Can you work these out from the model? Positions are in its coordinate system, mm. Face numbers are marked on the shaded views. Coordinates: 2 decimals unless noted, no trailing zeros. Loops run counter-clockwise (first coordinate to the right, second up) from the corner with the lowest first, then second, coordinate; pieces in that order, holes last.
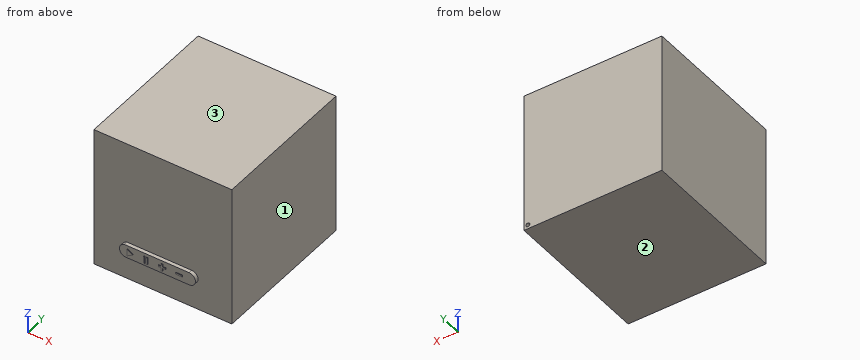
```python
from build123d import *

# Parameters (mm, degrees)
F0_W      = 93.715839088
F0_H      = 96.0587337613
F1_DEPTH  = 101.6
F2_W      = 8.2945693284
F2_H      = 8.6991842836
F2_W_2    = 8.0922637135
F2_W_3    = 8.2945674658
F2_W_4    = 7.8899562359
F3_DEPTH  = 2.54
F5_DEPTH  = 3
F6_W      = 0.9676124901
F6_H      = 4.834022373
F6_W_2    = 0.8269865066
F7_DEPTH  = 0.5
F8_W      = 1.12604897
F8_H      = 4.834022373
F9_DEPTH  = 0.5
F10_W     = 4.8627895303
F10_H     = 1.0272618383
F11_DEPTH = 0.5
F12_W     = 4.4415825978
F12_H     = 1.0272618383
F13_DEPTH = 0.5
F14_R     = 1.3332383726
F15_DEPTH = 6.35
F16_R     = 0.5696263833
F17_DEPTH = 7.62


with BuildPart() as f1:
    # F0 (on Front) → F1 (new body)
    with BuildSketch(Plane.XZ):
        with Locations((-0.6508044899, 1.3016089797)):
            Rectangle(F0_W, F0_H)
    extrude(amount=F1_DEPTH)

    # F2 (on face) → F3 (join)
    with BuildSketch(Plane.XZ.offset(101.6)):
        with BuildLine():
            Line((-19.5664688945, -20.8509583026), (-25.2310521901, -20.8509583026))
            ThreePointArc((-25.2310521901, -20.8509583026), (-28.4223170669, -25.358390925), (-24.8264390975, -29.5501425862))
            Line((-24.8264390975, -29.5501425862), (-19.5664688945, -29.5501425862))
            Line((-19.5664688945, -29.5501425862), (-19.5664688945, -20.8509583026))
        make_face()
        with Locations((-15.4191842303, -25.2005504444)):
            Rectangle(F2_W, F2_H)
        with Locations((-7.2257677093, -25.2005504444)):
            Rectangle(F2_W_2, F2_H)
        with Locations((0.9676478803, -25.2005504444)):
            Rectangle(F2_W_3, F2_H)
        with Locations((9.0599097311, -25.2005504444)):
            Rectangle(F2_W_4, F2_H)
        with BuildLine():
            Line((18.8717804849, -20.8509583026), (13.0048878491, -20.8509583026))
            Line((13.0048878491, -20.8509583026), (13.0048878491, -29.5501425862))
            Line((13.0048878491, -29.5501425862), (18.8717804849, -29.5501425862))
            ThreePointArc((18.8717804849, -29.5501425862), (23.2213726267, -25.2005504444), (18.8717804849, -20.8509583026))
        make_face()
    extrude(amount=F3_DEPTH)

    # F4 (on face) → F5 (join)
    with BuildSketch(Plane.XZ.offset(101.6)):
        Polygon((-19.0216936171, -25.3522377461), (-22.935193032, -22.9352265596), (-22.935193032, -27.7692489326), align=None)
    extrude(amount=F5_DEPTH)

    # F6 (on face) → F7 (join)
    with BuildSketch(Plane.XZ.offset(104.14)):
        with Locations((-11.4101376384, -25.3522377461)):
            Rectangle(F6_W, F6_H)
        with Locations((-9.6004614606, -25.3522377461)):
            Rectangle(F6_W_2, F6_H)
    extrude(amount=F7_DEPTH)

    # F8 (on face) → F9 (join)
    with BuildSketch(Plane.XZ.offset(104.14)):
        with Locations((0.563024485, -25.3522377461)):
            Rectangle(F8_W, F8_H)
    extrude(amount=F9_DEPTH)

    # F10 (on face) → F11 (join)
    with BuildSketch(Plane.XZ.offset(104.14)):
        with Locations((0.7227337919, -25.1438906416)):
            Rectangle(F10_W, F10_H)
    extrude(amount=F11_DEPTH)

    # F12 (on face) → F13 (join)
    with BuildSketch(Plane.XZ.offset(104.14)):
        with Locations((12.3583828099, -25.1438906416)):
            Rectangle(F12_W, F12_H)
    extrude(amount=F13_DEPTH)

    # F14 (on face) → F15 (cut)
    with BuildSketch(Plane(origin=(0, 0, 0), x_dir=(-1, 0, 0), z_dir=(0, 1, 0))):
        with Locations((-43.6146184802, -43.905235827)):
            Circle(F14_R)
    extrude(amount=-F15_DEPTH, mode=Mode.SUBTRACT)

    # F16 (on face) → F17 (cut)
    with BuildSketch(Plane(origin=(0, 0, 0), x_dir=(-1, 0, 0), z_dir=(0, 1, 0))):
        with Locations((-43.6146184802, -43.905235827)):
            Circle(F16_R)
    extrude(amount=-F17_DEPTH, mode=Mode.SUBTRACT)


solid = f1.part
```
(1) I want a section at C-C on x = -34.5. Write out the boundary of the cut face in (y, z), then the cut area to 3 significant figures.
Check values:
outline: (-101.6, -46.73) - (0, -46.73) - (0, 49.33) - (-101.6, 49.33) - close
area: 9,760 mm2
(2) If we mould it in two halves opening along Z, with no side actions, what happens to the marked faces 1, 2 and 3? For each: released by +Z, released by -Z, zero draft, split by the parting line, or undercut.
Check values:
face 1: zero draft
face 2: released by -Z
face 3: released by +Z
(3) I'm going to push flat-ended pins straight in: pin 1 (12 mm diameter, centred on x = 7.5, z = 30, fed in from -Y); pin 2 (3 mm diameter, centred on x = -4.5, y = -102.5, fed in from +Z); pin 3 (0.8 mm diameter, centred on x = 44, z = -44, fed in from +Y); pin 4 (0.6 mm diameter, centred on x = -0.5, y = -104.5, fed in from +Z). Where does each tip first touch, or does it pass through?
Check values:
pin 1: stops at y = -101.6
pin 2: stops at z = 49.33
pin 3: stops at y = -6.35
pin 4: stops at z = -24.63
(4) I want a section at B-B on z = -3.5. Write out the boundary of the cut face in (x, y).
Check values:
outline: (-47.51, -101.6) - (46.21, -101.6) - (46.21, 0) - (-47.51, 0) - close
(5) I want a section at A-A on x = 5.5. Write out the boundary of the cut face in (y, z), then the cut area to 3 significant figures.
Check values:
outline: (-104.14, -29.55) - (-101.6, -29.55) - (-101.6, -46.73) - (0, -46.73) - (0, 49.33) - (-101.6, 49.33) - (-101.6, -20.85) - (-104.14, -20.85) - close
area: 9,780 mm2
(6) If I drill on probe 1 along Y at (x, z) = (5.5, -2); probe 2 along Y at (x, z) = (-19, -26), over which ranges is the centre line in solid material (lowest first)?
Check values:
probe 1: y = -101.6 to 0
probe 2: y = -104.14 to 0
